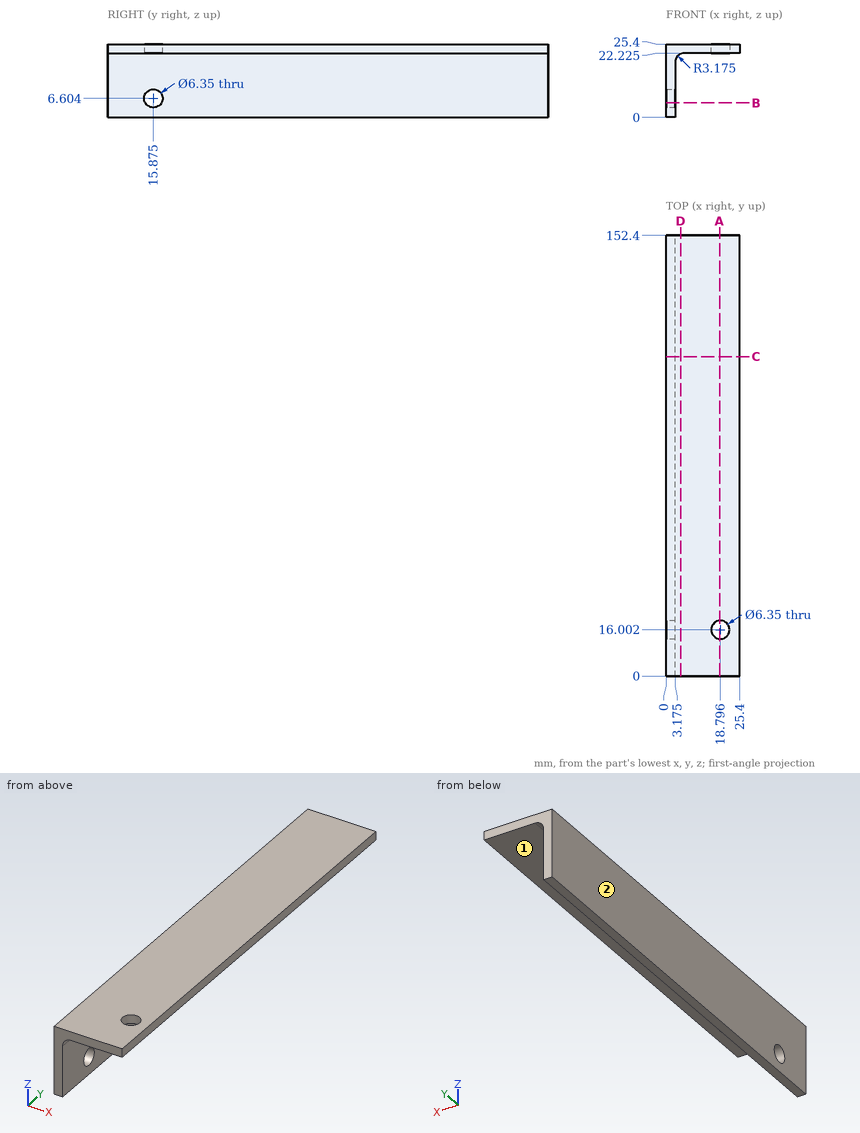
For this review, use the dimensioned drawing (mm, ordinates from the lowest corner) and the shaded views. A direction names the side the tool comes from. Give positions to 0.01 mm unless a question says otherwise; leave off trailing zeros. Order: outer loops, then holes, each group sorted by start corner. A loop starts at its lowest first (then second) coordinate and runs counter-clockwise, first axis right, second up. Notation, with made-up numbers: (38.5, 84.25) - (49.5, 84.25) arc R31 cw to (49.5, 116.25) - close; hole circle Ø6 at (16, 72). An arc over 180 degrees is marked (long way). Write item = value, one per line. Start each with the question number.
Q1. To check wall thickness, follow L1, parallel to Z at x = 23.5, y = 139 (3 decimals); L2, parallel to X at y = 19, z = 1.25 (3 decimals); L3, parallel to Y at x = 18.5, z = 22.75. State the ranges of each line that lie inside material, in increasing order. Write a range as from..to.
Q2. Tool access review of the marked faces 1 and 2: name each direction out of +Z, -Z, +X, -X, +Y, -Y from which nothing blocks a thin tool from reaching the whole face with its end or side.
Q3. We need section C-C on y = 110.5. State the section outline as (x, z) points (3 decimals), plus the area to 3 significant figures.
Q4. We need section D-D on x = 5. State the section outline as (y, z) points.
Q5. We need section B-B on z = 5. State the section outline as (x, y) points (3 decimals), plus the area to 3 significant figures.
Q6. We need section A-A on x = 18.5. State the section outline as (y, z) points (3 decimals).
Q7. Clearance check with a flat-ended pin moving along its axis: pin 1 Ø2 at (y, z) = (127, 4.5) entering from +X (3 decimals). State where the tip first meets the part, or that it passes through.
Working result:
q1.L1 = 22.225..25.4
q1.L2 = 0..3.175
q1.L3 = 0..12.84, 19.16..152.4
q2.face_1 = -Z, +X, +Y, -Y
q2.face_2 = +Z, -Z, -X, +Y, -Y
q3.outline = (0, 0) - (3.175, 0) - (3.175, 19.05) arc R3.175 cw to (6.35, 22.225) - (25.4, 22.225) - (25.4, 25.4) - (0, 25.4) - close
q3.area = 153 mm²
q4.outline = (0, 21.92) - (152.4, 21.92) - (152.4, 25.4) - (0, 25.4) - close
q5.outline = (0, 0) - (3.175, 0) - (3.175, 13.135) - (0, 13.135) - close; (0, 18.615) - (3.175, 18.615) - (3.175, 152.4) - (0, 152.4) - close
q5.area = 466 mm²
q6.outline = (0, 22.225) - (12.841, 22.225) - (12.841, 25.4) - (0, 25.4) - close; (19.163, 22.225) - (152.4, 22.225) - (152.4, 25.4) - (19.163, 25.4) - close
q7.pin_1 = 3.175
